```python
from build123d import *

# Parameters (mm, degrees)
SKETCH_1_W      = 50
SKETCH_1_H      = 50
EXTRUDE_1_DEPTH = 3
SKETCH_2_W      = 50
SKETCH_2_H      = 50
SKETCH_2_W_2    = 44
SKETCH_2_H_2    = 44
EXTRUDE_2_DEPTH = 27
SKETCH_3_W      = 4
SKETCH_3_H      = 1.5
SKETCH_3_W_2    = 1.5
SKETCH_3_H_2    = 4
EXTRUDE_3_DEPTH = 4


with BuildPart() as part:
    # 草图1 → 凸台-拉伸1 (new body)
    with BuildSketch(Plane(origin=(0, 0, 0), x_dir=(1, 0, 0), z_dir=(0, 1, 0))):
        Rectangle(SKETCH_1_W, SKETCH_1_H)
    extrude(amount=EXTRUDE_1_DEPTH)

    # 草图2 → 凸台-拉伸2 (add)
    with BuildSketch(Plane(origin=(0, 3, 0), x_dir=(1, 0, 0), z_dir=(0, 1, 0))):
        Rectangle(SKETCH_2_W, SKETCH_2_H)
        Rectangle(SKETCH_2_W_2, SKETCH_2_H_2, mode=Mode.SUBTRACT)
    extrude(amount=EXTRUDE_2_DEPTH)

    # 草图3 → 凸台-拉伸3 (add)
    with BuildSketch(Plane(origin=(0, 30, 0), x_dir=(1, 0, 0), z_dir=(0, 1, 0))):
        with Locations((-8, -22.75)):
            Rectangle(SKETCH_3_W, SKETCH_3_H)
        with Locations((8, -22.75)):
            Rectangle(SKETCH_3_W, SKETCH_3_H)
        with Locations((-22.75, 8)):
            Rectangle(SKETCH_3_W_2, SKETCH_3_H_2)
        with Locations((-22.75, -8)):
            Rectangle(SKETCH_3_W_2, SKETCH_3_H_2)
        with Locations((8, 22.75)):
            Rectangle(SKETCH_3_W, SKETCH_3_H)
        with Locations((-8, 22.75)):
            Rectangle(SKETCH_3_W, SKETCH_3_H)
        with Locations((22.75, -8)):
            Rectangle(SKETCH_3_W_2, SKETCH_3_H_2)
        with Locations((22.75, 8)):
            Rectangle(SKETCH_3_W_2, SKETCH_3_H_2)
    extrude(amount=EXTRUDE_3_DEPTH)

    # 草图4 → 放样2 section 0
    with BuildSketch(Plane(origin=(0, 34, 0), x_dir=(1, 0, 0), z_dir=(0, 1, 0))):
        with BuildLine():
            Line((-23.5, 10), (-23.6, 10))
            Line((-23.6, 10), (-23.6, 6))
            Line((-23.6, 6), (-23.5, 6))
            Line((-23.5, 6), (-23.5, 10))
        make_face()
    # 草图6 → 放样2 section 1
    with BuildSketch(Plane(origin=(0, 32, 0), x_dir=(1, 0, 0), z_dir=(0, 1, 0))):
        with BuildLine():
            Line((-23.5, 10), (-25, 10))
            Line((-25, 10), (-25, 6))
            Line((-25, 6), (-23.5, 6))
            Line((-23.5, 6), (-23.5, 10))
        make_face()
    loft()

    # 草图8 → 放样3 section 0
    with BuildSketch(Plane(origin=(0, 34, 0), x_dir=(1, 0, 0), z_dir=(0, 1, 0))):
        with BuildLine():
            Line((-23.5, -6), (-23.6, -6))
            Line((-23.6, -6), (-23.6, -10))
            Line((-23.6, -10), (-23.5, -10))
            Line((-23.5, -10), (-23.5, -6))
        make_face()
    # 草图9 → 放样3 section 1
    with BuildSketch(Plane(origin=(0, 32, 0), x_dir=(1, 0, 0), z_dir=(0, 1, 0))):
        with BuildLine():
            Line((-23.5, -6), (-25, -6))
            Line((-25, -6), (-25, -10))
            Line((-25, -10), (-23.5, -10))
            Line((-23.5, -10), (-23.5, -6))
        make_face()
    loft()

    # 草图10 → 放样4 section 0
    with BuildSketch(Plane(origin=(0, 34, 0), x_dir=(1, 0, 0), z_dir=(0, 1, 0))):
        with BuildLine():
            Line((-10, -23.5), (-6, -23.5))
            Line((-6, -23.5), (-6, -23.6))
            Line((-6, -23.6), (-10, -23.6))
            Line((-10, -23.6), (-10, -23.5))
        make_face()
    # 草图11 → 放样4 section 1
    with BuildSketch(Plane(origin=(0, 32, 0), x_dir=(1, 0, 0), z_dir=(0, 1, 0))):
        with BuildLine():
            Line((-10, -23.5), (-6, -23.5))
            Line((-6, -23.5), (-6, -25))
            Line((-6, -25), (-10, -25))
            Line((-10, -25), (-10, -23.5))
        make_face()
    loft()

    # 草图12 → 放样5 section 0
    with BuildSketch(Plane(origin=(0, 34, 0), x_dir=(1, 0, 0), z_dir=(0, 1, 0))):
        with BuildLine():
            Line((6, -23.5), (10, -23.5))
            Line((10, -23.5), (10, -23.6))
            Line((10, -23.6), (6, -23.6))
            Line((6, -23.6), (6, -23.5))
        make_face()
    # 草图13 → 放样5 section 1
    with BuildSketch(Plane(origin=(0, 32, 0), x_dir=(1, 0, 0), z_dir=(0, 1, 0))):
        with BuildLine():
            Line((6, -23.5), (10, -23.5))
            Line((10, -23.5), (10, -25))
            Line((10, -25), (6, -25))
            Line((6, -25), (6, -23.5))
        make_face()
    loft()

    # 草图14 → 放样6 section 0
    with BuildSketch(Plane(origin=(0, 34, 0), x_dir=(1, 0, 0), z_dir=(0, 1, 0))):
        with BuildLine():
            Line((23.5, -10), (23.6, -10))
            Line((23.6, -10), (23.6, -6))
            Line((23.6, -6), (23.5, -6))
            Line((23.5, -6), (23.5, -10))
        make_face()
    # 草图15 → 放样6 section 1
    with BuildSketch(Plane(origin=(0, 32, 0), x_dir=(1, 0, 0), z_dir=(0, 1, 0))):
        with BuildLine():
            Line((23.5, -10), (25, -10))
            Line((25, -10), (25, -6))
            Line((25, -6), (23.5, -6))
            Line((23.5, -6), (23.5, -10))
        make_face()
    loft()

    # 草图16 → 放样7 section 0
    with BuildSketch(Plane(origin=(0, 34, 0), x_dir=(1, 0, 0), z_dir=(0, 1, 0))):
        with BuildLine():
            Line((23.5, 6), (23.6, 6))
            Line((23.6, 6), (23.6, 10))
            Line((23.6, 10), (23.5, 10))
            Line((23.5, 10), (23.5, 6))
        make_face()
    # 草图17 → 放样7 section 1
    with BuildSketch(Plane(origin=(0, 32, 0), x_dir=(1, 0, 0), z_dir=(0, 1, 0))):
        with BuildLine():
            Line((23.5, 6), (25, 6))
            Line((25, 6), (25, 10))
            Line((25, 10), (23.5, 10))
            Line((23.5, 10), (23.5, 6))
        make_face()
    loft()

    # 草图18 → 放样8 section 0
    with BuildSketch(Plane(origin=(0, 34, 0), x_dir=(1, 0, 0), z_dir=(0, 1, 0))):
        with BuildLine():
            Line((-6, 23.5), (-10, 23.5))
            Line((-10, 23.5), (-10, 23.6))
            Line((-10, 23.6), (-6, 23.6))
            Line((-6, 23.6), (-6, 23.5))
        make_face()
    # 草图19 → 放样8 section 1
    with BuildSketch(Plane(origin=(0, 32, 0), x_dir=(1, 0, 0), z_dir=(0, 1, 0))):
        with BuildLine():
            Line((-6, 23.5), (-10, 23.5))
            Line((-10, 23.5), (-10, 25))
            Line((-10, 25), (-6, 25))
            Line((-6, 25), (-6, 23.5))
        make_face()
    loft()

    # 草图20 → 放样9 section 0
    with BuildSketch(Plane(origin=(0, 34, 0), x_dir=(1, 0, 0), z_dir=(0, 1, 0))):
        with BuildLine():
            Line((10, 23.5), (6, 23.5))
            Line((6, 23.5), (6, 23.6))
            Line((6, 23.6), (10, 23.6))
            Line((10, 23.6), (10, 23.5))
        make_face()
    # 草图21 → 放样9 section 1
    with BuildSketch(Plane(origin=(0, 32, 0), x_dir=(1, 0, 0), z_dir=(0, 1, 0))):
        with BuildLine():
            Line((10, 23.5), (6, 23.5))
            Line((6, 23.5), (6, 25))
            Line((6, 25), (10, 25))
            Line((10, 25), (10, 23.5))
        make_face()
    loft()


solid = part.part
```
The model under review builds one solid part; all positions refer to its coordinate system, in mm. A direction names the side the tool comes from. Give positions to 0.01 mm unless a question says otherwise; leave off trailing zeros. Order: outer loops, then holes, each group sorted by start corner. A loop starts at its lowest first (then second) coordinate and runs counter-clockwise, first axis right, second up. Notation, with made-up numbers: (81.25, 37.25) - (115.25, 37.25) arc R14 ccw to (115.25, 45.25) - close; hole circle Ø2 at (-29, -31.5). An arc over 180 degrees is marked (long way). Use CSV: the item, a comma, the result in double quotes. Start each with the question number.
Q1. Tool access review of faces 1 (the flat face through (24, 32, -8)), 2 (the flat face through (-23, 32, 6)), 3 (the flat face through (6, 32, 23)), 4 (the flat face through (-10, 32, -23)), 5 (the flat face through (23, 32, -10)): name each direction out of +Z, -Z, +X, -X, +Y, -Y from which nothing blocks a thin tool from reaching the whole face with its end or side.
Q2. We need section D-D, the plane x = -2. Write out the cut boundary in (y, z).
Q3. Clearance check with flat-ended pins moving along their axes: pin 1 Ø2.5 at (y, z) = (32, 24) entering from -X; pin 2 Ø1.2 at (x, z) = (-24, 8) entering from -Y; pin 3 Ø0.6 at (x, y) = (8, 31) entering from -Z; pin 4 Ø1 at (x, y) = (8.5, 31) entering from +Z. State where each tip first meets the part, or that it passes through.
Q4. To check wall thickness, follow line 1 along Z through (x, y) = (-12, 8); line 2 along Y through (x, z) = (20, -1). State the ranges of each line that lie inside material, in increasing order. Write a range as [from, to].
Q5. We need section C-C, the plane z = 7. Write out the cut boundary in (x, y).
Q6. We need section B-B, the plane y = 10. Write out the cut boundary in (x, z).
Q7. The part is to be moulded in two halves that separate along Y. For faces 6 (the flat face through (-23.5, 31, -8)), 7 (the flat face through (-23, 32, -6)), 8 (the flat face through (8, 34, 23)), say which applies: +Y half, -Y half, draft (parallel to the pull), parting line (faces both ways), or undercut.
Q8. We need section A-A, the plane x = -9. Write out the cut boundary in (y, z), and give its area (3 significant figures).
Outcome:
1,face 1,"+Z, -Z, +X"
1,face 2,"+X, -X, +Y"
1,face 3,"+Z, -Z, +Y"
1,face 4,"+Z, -Z, -X, +Y"
1,face 5,"-Z, +X, -X, +Y"
2,outline,"(0, -25) - (30, -25) - (30, -22) - (3, -22) - (3, 22) - (30, 22) - (30, 25) - (0, 25) - close"
3,pin 1,"stops at x = -10"
3,pin 2,"stops at y = 0"
3,pin 3,"stops at z = -23.5"
3,pin 4,"stops at z = 23.5"
4,line 1,"z = [-25, -22], [22, 25]"
4,line 2,"y = [0, 3]"
5,outline,"(-25, 0) - (25, 0) - (25, 30) - (23.5, 30) - (23.5, 32) - (25, 32) - (23.6, 34) - (22, 34) - (22, 3) - (-22, 3) - (-22, 34) - (-23.6, 34) - (-25, 32) - (-23.5, 32) - (-23.5, 30) - (-25, 30) - close"
6,outline,"(-25, -25) - (25, -25) - (25, 25) - (-25, 25) - close; hole (-22, -22) - (22, -22) - (22, 22) - (-22, 22) - close"
7,face 6,"undercut"
7,face 7,"draft"
7,face 8,"+Y half"
8,outline,"(0, -25) - (30, -25) - (30, -23.5) - (32, -23.5) - (32, -25) - (34, -23.6) - (34, -22) - (3, -22) - (3, 22) - (34, 22) - (34, 23.6) - (32, 25) - (32, 23.5) - (30, 23.5) - (30, 25) - (0, 25) - close"
8,area,"327 mm^2"
